Geometry: final body of the model. Coordinates: model frame, mm. A direction names the side the tool comes from. Give positions to 0.01 mm unless a question says otherwise; leave off trailing zeros. Order: outer loops, then holes, each group sorted by start corner. A loop starts at its lowest first (then second) coordinate and runs counter-clockwise, first axis right, second up. Notation, with made-up numbers: M 17.5,70 L 69.5,70 A31 ccw 69.5,102 Z; hole C -23.5,-28 d4. An arc over 180 degrees is marked long. One line per item, written item: value. Start each with the question number.
```python
from build123d import *

# Parameters (mm, degrees)
EXTRUDE_1_DEPTH = 70


with BuildPart() as part:
    # 草圖1 → 填料-伸長1 (new body)
    with BuildSketch(Plane(origin=(0, 0, 0), x_dir=(1, 0, 0), z_dir=(0, 1, 0))):
        with BuildLine():
            Line((10.996587269, 18.037741282), (-45.487838574, -38.61479297))
            ThreePointArc((-45.487838574, -38.61479297), (-47.84934361, -38.895811815), (-49.888582931, -37.672218494))
            Line((-49.888582931, -37.672218494), (-52.721209644, -34.847997201))
            Line((-52.721209644, -34.847997201), (-54.839375613, -36.972467236))
            Line((-54.839375613, -36.972467236), (-52.0067489, -39.796688528))
            ThreePointArc((-52.0067489, -39.796688528), (-47.849605549, -41.783872953), (-43.363368539, -40.732958939))
            Line((-43.363368539, -40.732958939), (13.121057303, 15.919575313))
            ThreePointArc((13.121057303, 15.919575313), (15.009846467, 17.808364477), (16.898635631, 15.919575313))
            Line((16.898635631, 15.919575313), (49.482242531, -40.323722611))
            ThreePointArc((49.482242531, -40.323722611), (55.349857539, -42.316518092), (60.91576552, -39.592402078))
            Line((60.91576552, -39.592402078), (62.241081291, -38.094557591))
            Line((62.241081291, -38.094557591), (59.994314562, -36.106583934))
            Line((59.994314562, -36.106583934), (58.66899879, -37.60442842))
            ThreePointArc((58.66899879, -37.60442842), (55.618475046, -39.540333545), (52.078087051, -38.819863831))
            Line((52.078087051, -38.819863831), (19.494480151, 17.423434093))
            ThreePointArc((19.494480151, 17.423434093), (15.47366289, 20.886366054), (10.996587269, 18.037741282))
        make_face()
    extrude(amount=EXTRUDE_1_DEPTH)


solid = part.part
```
Q1. Mould query, pull axis X, two halves, no side actions, for faces 1 (the face through (-53.443, 34.51, 38.365)), 2 (the face through (-47.82, 34.51, 38.9)), 3 (the face through (-5, 70, 1)). Classes: +X half, -X half, draft (parallel to the pull), parting line (faces both ways), or undercut.
Q2. Section query B-B on y = 49.5. Return loops of the section in (x, z), and give its area (3 significant figures).
Q3. Section query D-D on x = 44.5. Return loops of the section in (y, z), and give its area (3 significant figures).
Q4. Section query C-C on x = 14.5. Return loops of the section in (y, z), and give its area (3 significant figures).
Q5. Contact query for flat-ended pins moving along their axis: pin 1 (4 mm diameter, centred on y = 60.5, z = -5, fed in from -X); pin 2 (6 mm diameter, centred on x = -33.5, y = 28.5, fed in from +Z); pin 3 (10 mm diameter, centred on y = 46, z = 11, fed in from +X); pin 4 (10 mm diameter, centred on x = 38.5, z = -0.5, fed in from +Y). Output: stop coordinate, or through.
Q6. Ray query, line 1 along X through (y, z) = (52.5, 35.5); line 2 along X through (y, z) = (27.5, 27); line 3 along X through (y, z) = (61.5, -2.5). Return the intervals inside material, ascending. Write a range as [from, to].
Q7. Section query A-A on z = 7.5. Return loops of the section in (x, y), and give its area (3 significant figures).
Q8. Set-up query: faces 4 (the face through (32.962, 34.51, 11.808)), 5 (the face through (-51.285, 34.51, 36.28)), 6 (the face through (-5, 0, 1)). Return all of +Z, -Z, +X, -X, +Y, -Y with unobstructed straight access to the full face (end or side cutting, diameter ignored); none if empty.
Results below:
1. face 1: -X half
1. face 2: undercut
1. face 3: draft
2. outline: M -54.84,36.97 L -52.72,34.85 L -49.89,37.67 A3.68 cw -45.49,38.61 L 11,-18.04 A4.45 ccw 19.49,-17.42 L 52.08,38.82 A4.83 cw 58.67,37.6 L 59.99,36.11 L 62.24,38.09 L 60.92,39.59 A8.12 ccw 49.48,40.32 L 16.9,-15.92 A1.89 cw 13.12,-15.92 L -43.36,40.73 A6.95 ccw -52.01,39.8 Z
2. area: 527 mm2
3. outline: M 0,25.74 L 70,25.74 L 70,31.72 L 0,31.72 Z
3. area: 419 mm2
4. outline: M 0,-20.85 L 70,-20.85 L 70,-17.74 L 0,-17.74 Z
4. area: 218 mm2
5. pin 1: x = -4
5. pin 2: z = 33.85
5. pin 3: x = 38.86
5. pin 4: through
6. line 1: [-53.37, -52.07], [-42.38, -38.15], [46.69, 50.15]
6. line 2: [-33.91, -29.67], [41.76, 45.23]
6. line 3: [-4.5, -0.26], [24.67, 28.14]
7. outline: M -14.47,0 L -10.23,0 L -10.23,70 L -14.47,70 Z; M 30.47,0 L 33.93,0 L 33.93,70 L 30.47,70 Z
7. area: 539 mm2
8. face 4: +Z, +Y, -Y
8. face 5: -Z, +Y, -Y
8. face 6: +Z, -Z, +X, -X, -Y
